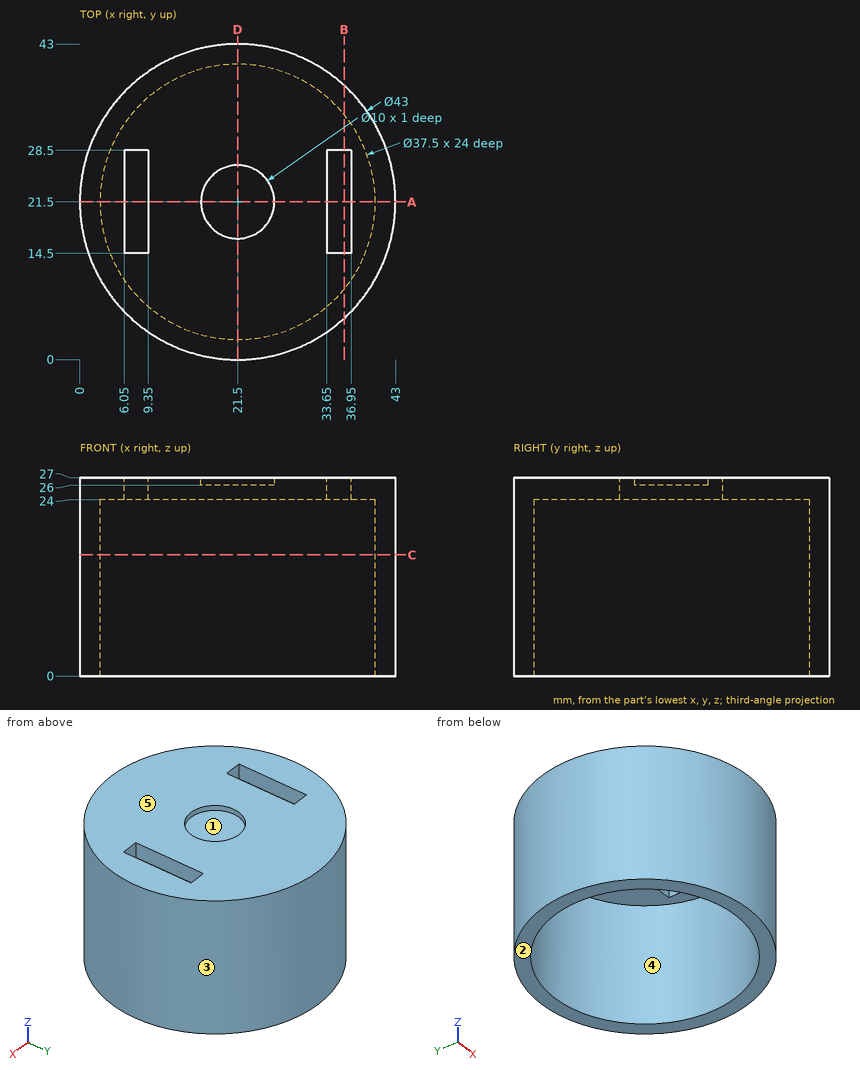
Check sheet for the drawn part. Datum: minimum x, y, z corner. Units: mm. A direction names the side the tool comes from. Round coordinates to 2 decimals unless told otherwise and drop trailing zeros. Write each loop counter-clockwise with the first axis right and the second up, starting at its lowest first coordinate (ties: lowest second). Pieces come first, ordered by that corner, then holes. Notation, with made-up numbers: (65, 3.5) - (86, 3.5) arc R18 cw to (86, 34.5) - close; hole circle Ø11 at (-32, 33). An arc over 180 degrees is marked (long way). Return JSON: item names as keys, results as strings.
Q1. Cross-section at A-A (y = 21.5). Record the boundary of the cut face in (x, z), then the cut area to 3 significant figures.
Returned:
{"outline": "(0, 0) - (2.75, 0) - (2.75, 24) - (6.05, 24) - (6.05, 27) - (0, 27) - close; (9.35, 24) - (33.65, 24) - (33.65, 27) - (26.5, 27) - (26.5, 26) - (16.5, 26) - (16.5, 27) - (9.35, 27) - close; (36.95, 24) - (40.25, 24) - (40.25, 0) - (43, 0) - (43, 27) - (36.95, 27) - close", "area": "231 mm²"}
Q2. Access from +Z, -Z, +X, -X, +Y, -Y to the whole of each face (thin tool, end or side, straight path). Record for the marked faces 4 and 5.
Returned:
{"face 4": "-Z", "face 5": "+Z, +X, -X, +Y, -Y"}
Q3. Cross-section at C-C (z = 16.5). Record the boundary of the cut face in (x, y).
Returned:
{"outline": "circle Ø43 at (21.5, 21.5); hole circle Ø37.5 at (21.5, 21.5)"}
Q4. Depth check by flat-ended pin: P1, Ø8, axis at x = 21.5, y = 21.5, coming from the -Z side; P2, Ø0.9, axis at y = 19.5, z = 25, coming from the +X side; P3, Ø10, axis at x = 26.5, z = 20, coming from the -Y side. Enter the tip coordinate at first touch or a pass-through.
Returned:
{"P1": "stops at z = 24", "P2": "stops at x = 42.94", "P3": "stops at y = 0"}
Q5. Cross-section at B-B (x = 36). Record the boundary of the cut face in (y, z).
Returned:
{"outline": "(5.63, 0) - (9.61, 0) - (9.61, 24) - (14.5, 24) - (14.5, 27) - (5.63, 27) - close; (28.5, 24) - (33.39, 24) - (33.39, 0) - (37.37, 0) - (37.37, 27) - (28.5, 27) - close"}
Q6. Draft check along X on the marked faces 1, 2 and 3. Enter one of: released by +X, released by -X, zero draft, split by the parting line, or undercut.
Returned:
{"face 1": "undercut", "face 2": "zero draft", "face 3": "split by the parting line"}
Q7. Cross-section at D-D (x = 21.5). Record the boundary of the cut face in (y, z), then the cut area to 3 significant figures.
Returned:
{"outline": "(0, 0) - (2.75, 0) - (2.75, 24) - (40.25, 24) - (40.25, 0) - (43, 0) - (43, 27) - (26.5, 27) - (26.5, 26) - (16.5, 26) - (16.5, 27) - (0, 27) - close", "area": "251 mm²"}
Q8. Scan lines: L1, parallel to Y at x = 21.5, z = 26.3; L2, parallel to X at y = 22, z = 15.25; L3, parallel to Z at x = 32, y = 12.5. Record each from-to range of solid material in increasing order. Write a range as from..to.
Returned:
{"L1": "y = 0..16.5, 26.5..43", "L2": "x = 0.01..2.76, 40.24..42.99", "L3": "z = 24..27"}
